Answer from the drawing. Dimensions are ordinates in mm from the lowest x, y and z of the part. A direction names the side the tool comes from. Coordinates: 2 decimals unless noted, no trailing zeros. Write each loop counter-clockwise with the first axis right and the second up, starting at its lowest first coordinate (ties: lowest second). Pieces come first, ordered by that corner, then holes.
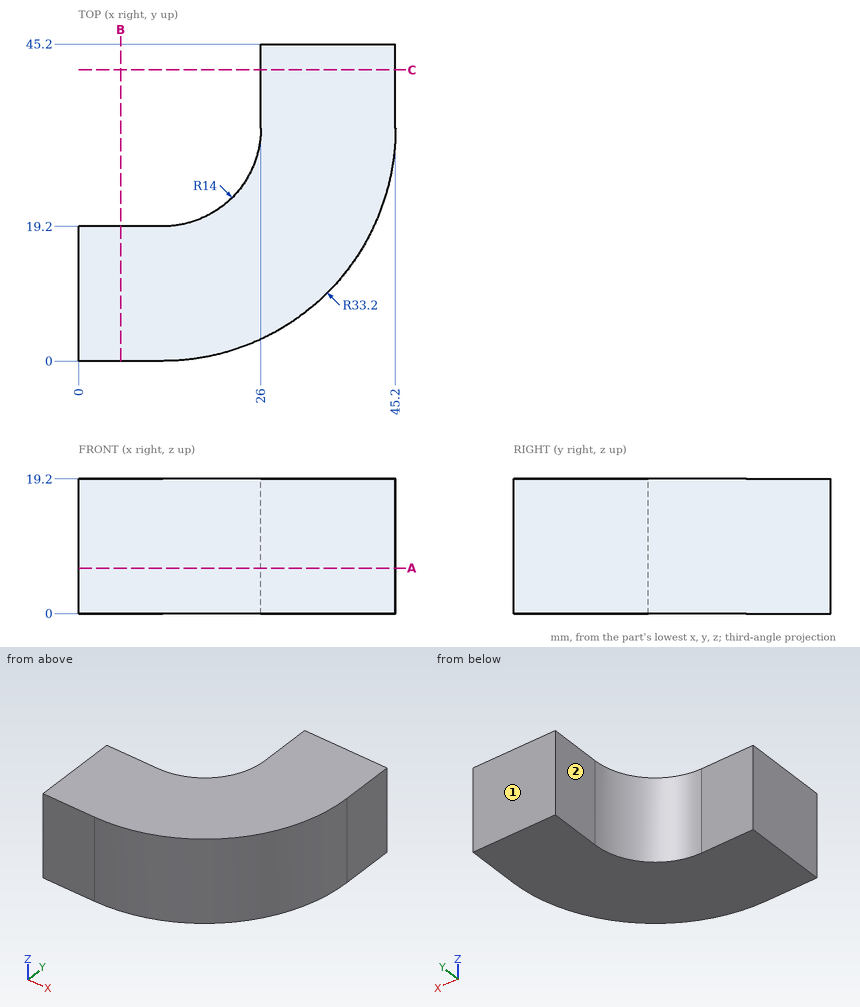
(1) Which of the six approach directions +Z, -Z, +X, -X, +Y, -Y give full straight-line access (tool end or side, diameter ignored) to the marked faces 1 and 2?
(2) Section A-A, the plane z = 6.5 is taken. Write down the section's boundary in (x, y), plus the area to 3 significant figures.
(3) Section C-C, the plane y = 41.5 is taken. Write down the section's boundary in (x, z), plus the area to 3 significant figures.
(4) Find the intervals of material crossed by probe 1 along X at (y, z) = (36, 8.5); probe 2 along Y at (x, z) = (4.5, 12); probe 3 along Y at (x, z) = (36.5, 11.75), in increasing order.
(5) Section B-B, the plane x = 6 is taken. Write down the section's boundary in (y, z).
(6) Each of these flat-tipped pins is pushed along its axis until it touches: pin 1 (2 mm diameter, centred on y = 22, z = 4, fed in from +X); pin 2 (9.5 mm diameter, centred on y = 36.5, z = 8.5, fed in from -X); pin 3 (4 mm diameter, centred on x = 19, z = 13.5, fed in from +Y); pin 4 (2 mm diameter, centred on x = 13, y = 21.5, fed in from +Z). Where does it stop, or does it pass through?
Solution:
1. face 1: +Z, -Z, +X, -X, +Y
1. face 2: +Z, -Z, -X, +Y
2. outline: (0, 0) - (12, 0) arc R33.2 ccw to (45.2, 33.2) - (45.2, 45.2) - (26, 45.2) - (26, 33.2) arc R14 cw to (12, 19.2) - (0, 19.2) - close
2. area: 1,170 mm2
3. outline: (26, 0) - (45.2, 0) - (45.2, 19.2) - (26, 19.2) - close
3. area: 369 mm2
4. probe 1: x = 26 to 45.2
4. probe 2: y = 0 to 19.2
4. probe 3: y = 10.79 to 45.2
5. outline: (0, 0) - (19.2, 0) - (19.2, 19.2) - (0, 19.2) - close
6. pin 1: stops at x = 43.59
6. pin 2: stops at x = 25.92
6. pin 3: stops at y = 22.48
6. pin 4: passes through
